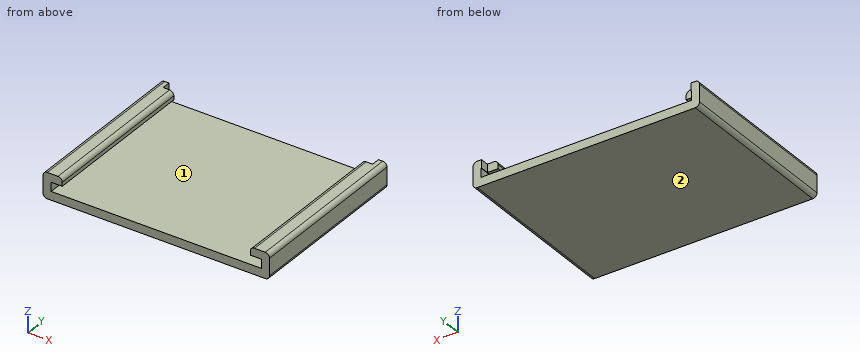
from build123d import *

# Parameters (mm, degrees)
BOSS_EXTRUDE1_DEPTH = 40
FILLET1_R           = 1
SKETCH3_W           = 3.059746362
SKETCH3_H           = 2.82490347
CUT_EXTRUDE1_DEPTH  = 2
SKETCH2_W           = 2.5
SKETCH2_H           = 2
SKETCH2_H_2         = 2.1
CUT_EXTRUDE2_DEPTH  = 45
SKETCH6_W           = 0.1
SKETCH6_H           = 2.1
CUT_EXTRUDE3_DEPTH  = 40


with BuildPart() as part:
    # Sketch1 → Boss-Extrude1 (new body)
    with BuildSketch(Plane(origin=(0, 0, 0), x_dir=(1, 0, 0), z_dir=(0, 1, 0))):
        Polygon((26.5, 2), (-26.5, 2), (-26.5, -4), (-22, -4), (-22, -2), (-24.5, -2), (-24.5, 0), (24.5, 0), (24.5, -2), (22, -2), (22, -4), (26.5, -4), align=None)
    extrude(amount=BOSS_EXTRUDE1_DEPTH)

    # Fillet1
    fillet1_edges = [part.edges().sort_by_distance(p)[0] for p in [
        (22, 20, 4),
        (26.5, 20, 4),
        (26.5, 20, -2),
        (-26.5, 20, -2),
        (-26.5, 20, 4),
        (-22, 20, 4),
    ]]
    fillet(fillet1_edges, radius=FILLET1_R)

    # Sketch3 → Cut-Extrude1 (cut)
    with BuildSketch(Plane(origin=(0, 40, 0), x_dir=(1, 0, 0), z_dir=(0, 1, 0))):
        Polygon((-24.5, -4.82490347), (-21.440253638, -4.82490347), (-21.343886973, -2.1), (-24.5, -2.1), align=None)
        with Locations((22.970126819, -3.412451735)):
            Rectangle(SKETCH3_W, SKETCH3_H)
    extrude(amount=-CUT_EXTRUDE1_DEPTH, mode=Mode.SUBTRACT)

    # Sketch2 → Cut-Extrude2 (cut)
    with BuildSketch(Plane(origin=(0, 0, 0), x_dir=(1, 0, 0), z_dir=(0, 1, 0))):
        with Locations((23.25, -1)):
            Rectangle(SKETCH2_W, SKETCH2_H)
        with Locations((-23.25, -1.05)):
            Rectangle(SKETCH2_W, SKETCH2_H_2)
    cut_extrude2 = extrude(amount=CUT_EXTRUDE2_DEPTH, mode=Mode.SUBTRACT)

    # Mirror1: Cut-Extrude2 across plane
    add(cut_extrude2.mirror(Plane(origin=(0, 0, 0), x_dir=(0, 0, 1), z_dir=(1, 0, 0))), mode=Mode.SUBTRACT)

    # Sketch6 → Cut-Extrude3 (cut)
    with BuildSketch(Plane(origin=(0, 40, 0), x_dir=(1, 0, 0), z_dir=(0, 1, 0))):
        with Locations((-24.55, -1.05)):
            Rectangle(SKETCH6_W, SKETCH6_H)
        with Locations((24.55, -1.05)):
            Rectangle(SKETCH6_W, SKETCH6_H)
    extrude(amount=-CUT_EXTRUDE3_DEPTH, mode=Mode.SUBTRACT)


solid = part.part
For this review, take the finished solid that the model builds, in its own axes (mm). Face numbers are marked on the shaded views. Give positions to 0.01 mm unless a question says otherwise; leave off trailing zeros. Order: outer loops, then holes, each group sorted by start corner. A loop starts at its lowest first (then second) coordinate and runs counter-clockwise, first axis right, second up. Notation, with made-up numbers: (12.25, 68.25) -> (27.25, 68.25) arc R15 ccw to (27.25, 88.25) -> close; hole circle Ø1 at (66.5, -15). An arc over 180 degrees is marked (long way). Write item = value, one per line.
1) To check wall thickness, follow L1, parallel to Z at x = -24, y = 32.5; L2, parallel to X at y = 37, z = 0.4; L3, parallel to Z at x = -6, y = 31. State the ranges of each line that lie inside material, in increasing order. Write a range as from..to.
Findings:
L1 = -2..0, 2.1..4
L2 = -26.5..-24.6, 24.6..26.5
L3 = -2..0
2) We need section B-B, the plane y = 33. Give the boundary of the cut face in (x, z).
Findings:
outline = (-26.5, -1) arc R1 ccw to (-25.5, -2) -> (25.5, -2) arc R1 ccw to (26.5, -1) -> (26.5, 3) arc R1 ccw to (25.5, 4) -> (23, 4) arc R1 ccw to (22, 3) -> (22, 2.1) -> (24.6, 2.1) -> (24.6, 0) -> (-24.6, 0) -> (-24.6, 2.1) -> (-22, 2.1) -> (-22, 3) arc R1 ccw to (-23, 4) -> (-25.5, 4) arc R1 ccw to (-26.5, 3) -> close
3) Draft analysis for pull direction X (two halves, no side actions). For the marked faces 1 and 2, state which applies: pulls with the +X half, pulls with the -X half, needs draft (parallel to the pull), parting line crosses it, or undercut.
Findings:
face_1 = undercut
face_2 = needs draft
4) We need section C-C, the plane x = 0.5. Give the boundary of the cut face in (y, z).
Findings:
outline = (0, -2) -> (40, -2) -> (40, 0) -> (0, 0) -> close
5) Insertion check: pin 1 (20 mm diameter, centred on x = 9, y = 15, fed in from +Z); pin 2 (3 mm diameter, centred on x = -5, z = 2.5, fed in from -Y). Each pin has a flat end and moves straight along its axis. Give the tip position at first contact, or say it passes through.
Findings:
pin_1 = 0
pin_2 = through
6) We need section A-A, the plane z = 1.55. Give the boundary of the cut face in (x, y), and give its area (3 significant figures).
Findings:
outline = (-26.5, 0) -> (-24.6, 0) -> (-24.6, 40) -> (-26.5, 40) -> close; (24.6, 0) -> (26.5, 0) -> (26.5, 40) -> (24.6, 40) -> close
area = 152 mm^2
